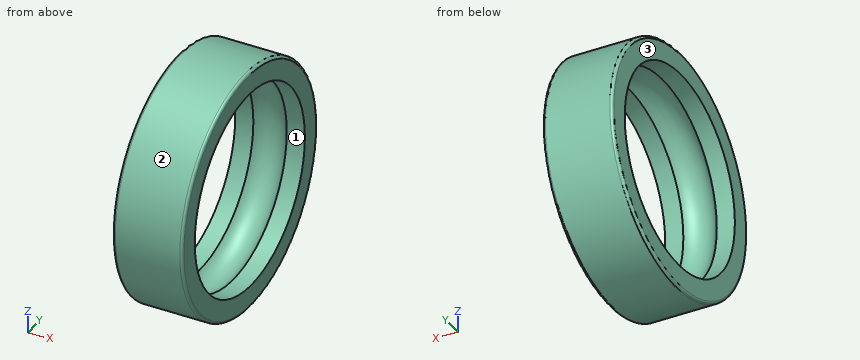
Autodesk Inventor part; units mm, degrees
ref_plane "dgbb_or_XY" through (0, 0, 0) normal (1, 0, 0) x (0, 0, -1)
ref_plane "dgbb_or_YZ" through (0, 0, 0) normal (0, 0, -1) x (0, 1, 0)
ref_plane "dgbb_or_ZX" through (0, 0, 0) normal (0, 1, 0) x (1, 0, 0)
sketch "Sketch_1" plane through (0, 0, 0) normal (0, 0, 1) x (1, 0, 0)
  line L0 (8, 0) -> (0, 0)
  line L1 (0, 11.44) -> (2.08, 11.44)
  arc A0 (5.92, 11.44) -> (2.08, 11.44) centre (4, 10) ccw
  line L2 (5.92, 11.44) -> (8, 11.44)
  line L3 (8, 11.44) -> (8, 13.7)
  arc A1 (8, 13.7) -> (7.7, 14) centre (7.7, 13.7) ccw
  line L4 (7.7, 14) -> (0.3, 14)
  arc A2 (0.3, 14) -> (0, 13.7) centre (0.3, 13.7) ccw
  line L5 (0, 13.7) -> (0, 11.44)
revolve "Revolution1" add sketch "Sketch_1" angle 360 about axis through (8, 0, 0) along (1, 0, 0)
ref_plane "dgbb_or_XY" through (0, 0, 0) normal (1, 0, 0) x (0, 0, -1)
ref_plane "dgbb_or_YZ" through (0, 0, 0) normal (0, 0, -1) x (0, 1, 0)
ref_plane "dgbb_or_ZX" through (0, 0, 0) normal (0, 1, 0) x (1, 0, 0)
ref_plane "dgbb_or1_XY" through (8, 0, 0) normal (1, 0, 0) x (0, 0, -1)
ref_plane "dgbb_or1_YZ" through (8, 0, 0) normal (0, 0, -1) x (0, 1, 0)
ref_plane "dgbb_or1_ZX" through (8, 0, 0) normal (0, 1, 0) x (1, 0, 0)
ref_plane "dgbb_or11_1_XY" through (4, 10, 0) normal (1, 0, 0) x (0, 0, -1)
ref_plane "dgbb_or11_1_YZ" through (4, 10, 0) normal (0, 0, -1) x (0, 1, 0)
ref_plane "dgbb_or11_1_ZX" through (4, 10, 0) normal (0, 1, 0) x (1, 0, 0)
ref_plane "dgbb_or11_2_XY" through (4, 6.2349, 7.8183) normal (1, 0, 0) x (0, 0, -1)
ref_plane "dgbb_or11_2_YZ" through (4, 6.2349, 7.8183) normal (0, 0, -1) x (0, 1, 0)
ref_plane "dgbb_or11_2_ZX" through (4, 6.2349, 7.8183) normal (0, 1, 0) x (1, 0, 0)
ref_plane "dgbb_or11_3_XY" through (4, -2.2252, 9.7493) normal (1, 0, 0) x (0, 0, -1)
ref_plane "dgbb_or11_3_YZ" through (4, -2.2252, 9.7493) normal (0, 0, -1) x (0, 1, 0)
ref_plane "dgbb_or11_3_ZX" through (4, -2.2252, 9.7493) normal (0, 1, 0) x (1, 0, 0)
ref_plane "dgbb_or11_4_XY" through (4, -9.0097, 4.3388) normal (1, 0, 0) x (0, 0, -1)
ref_plane "dgbb_or11_4_YZ" through (4, -9.0097, 4.3388) normal (0, 0, -1) x (0, 1, 0)
ref_plane "dgbb_or11_4_ZX" through (4, -9.0097, 4.3388) normal (0, 1, 0) x (1, 0, 0)
ref_plane "dgbb_or11_5_XY" through (4, -9.0097, -4.3388) normal (1, 0, 0) x (0, 0, -1)
ref_plane "dgbb_or11_5_YZ" through (4, -9.0097, -4.3388) normal (0, 0, -1) x (0, 1, 0)
ref_plane "dgbb_or11_5_ZX" through (4, -9.0097, -4.3388) normal (0, 1, 0) x (1, 0, 0)
ref_plane "dgbb_or11_6_XY" through (4, -2.2252, -9.7493) normal (1, 0, 0) x (0, 0, -1)
ref_plane "dgbb_or11_6_YZ" through (4, -2.2252, -9.7493) normal (0, 0, -1) x (0, 1, 0)
ref_plane "dgbb_or11_6_ZX" through (4, -2.2252, -9.7493) normal (0, 1, 0) x (1, 0, 0)
ref_plane "dgbb_or11_7_XY" through (4, 6.2349, -7.8183) normal (1, 0, 0) x (0, 0, -1)
ref_plane "dgbb_or11_7_YZ" through (4, 6.2349, -7.8183) normal (0, 0, -1) x (0, 1, 0)
ref_plane "dgbb_or11_7_ZX" through (4, 6.2349, -7.8183) normal (0, 1, 0) x (1, 0, 0)
properties part number "6001JRX Outer Ring"
Design review of the part built by this model. Coordinates are the model's own, in mm. Face numbers are marked on the shaded views. Coordinates: 2 decimals unless noted, no trailing zeros. Loops run counter-clockwise (first coordinate to the right, second up) from the corner with the lowest first, then second, coordinate; pieces in that order, holes last. Notation, with made-up numbers: (69.5, -23.75) -> (99.5, -23.75) arc R24 ccw to (99.5, -5.75) -> close; hole circle Ø5 at (-38.5, -2.75). An arc over 180 degrees is marked (long way). Use a Markdown table: item, result. Add a question column.
Item 1: Wall thickness on L1, parallel to Z at x = 1.2, y = 0; L2, parallel to Z at x = 4, y = -1.5; L3, parallel to X at y = -12, z = 6.75: over which ranges is each line inside the solid? List them lowest first. Write a range as from..to.
Item 2: We need section C-C, the plane x = 1.75. Write out the cut boundary in (y, z).
Item 3: We need section A-A, the plane y = 0. Write out the cut boundary in (x, z), and give its area (3 significant figures).
Item 4: The part is to be moulded in two halves that separate along Z. For the marked faces 1, 2 and 3, say which applies: +Z half, -Z half, draft (parallel to the pull), parting line (faces both ways), or undercut.
Item 5: Clearance check with a flat-ended pin moving along its axis: P1, Ø3, axis at x = 3, z = -3.5, coming from the +Y side. State where the tip first meets the part, or that it passes through.
Numbers:
| question | item | result |
|---|---|---|
| 1 | L1 | z = -14..-11.44, 11.44..14 |
| 1 | L2 | z = -13.92..-12.31, 12.31..13.92 |
| 1 | L3 | x = 0.01..7.99 |
| 2 | outline | circle Ø28 at (0, 0); hole circle Ø22.88 at (0, 0) |
| 3 | outline | (0, -13.7) arc R0.3 ccw to (0.3, -14) -> (7.7, -14) arc R0.3 ccw to (8, -13.7) -> (8, -11.44) -> (5.92, -11.44) arc R2.4 cw to (2.08, -11.44) -> (0, -11.44) -> close; (0, 11.44) -> (2.08, 11.44) arc R2.4 cw to (5.92, 11.44) -> (8, 11.44) -> (8, 13.7) arc R0.3 ccw to (7.7, 14) -> (0.3, 14) arc R0.3 ccw to (0, 13.7) -> close |
| 3 | area | 35.7 mm^2 |
| 4 | face 1 | undercut |
| 4 | face 2 | parting line |
| 4 | face 3 | draft |
| 5 | P1 | stops at y = 13.86 |
